Geometry check sheet. Reference: the model listing, model coordinates, mm. Coordinates: 2 decimals unless noted, no trailing zeros. Write each loop counter-clockwise with the first axis right and the second up, starting at its lowest first coordinate (ties: lowest second). Pieces come first, ordered by that corner, then holes. Notation, with made-up numbers: (-18.75, 76) -> (9.25, 76) arc R23 cw to (9.25, 102) -> close; hole circle Ø8 at (23.25, 11). An arc over 180 degrees is marked (long way). Put each result on its own line as item: value. Start each with the question number.
from build123d import *

# Parameters (mm, degrees)
F0_W        = 152.4
F0_H        = 101.6
F0_R        = 25.4
F1_DEPTH    = 76.2
F2_R        = 5.08
F3_R        = 5.08
F4_T1_DEPTH = 83.82
F4_S5_W     = 5.08
F4_S5_H     = 5.08
F4_T6_DEPTH = 5.08


# Not quite as in the source:
# - a fillet or chamfer that OpenCascade refuses, or shapes differently, is made with other operations: its cross-section is extruded or revolved along the edge and cut away or added


with BuildPart() as f1:
    # F0 (on Top) → F1 (new body)
    with BuildSketch(Plane.XY):
        Rectangle(F0_W, F0_H)
        Circle(F0_R, mode=Mode.SUBTRACT)
    extrude(amount=F1_DEPTH)

    # F2
    f2_edges = [f1.edges().sort_by_distance(p)[0] for p in [
        (-76.2, 0, 76.2),
    ]]
    fillet(f2_edges, radius=F2_R)

    # F3
    f3_edges = [f1.edges().sort_by_distance(p)[0] for p in [
        (2.54, 50.8, 76.2),
        (76.2, 0, 76.2),
        (2.54, -50.8, 76.2),
    ]]
    fillet(f3_edges, radius=F3_R)

    # F4: fillet of radius 5.08 on 1 edges, made by hand

    # F4_s2 → F4_t1 (cut)
    with BuildSketch(Plane.XY.offset(-12.7)):
        with BuildLine():
            ThreePointArc((76.2, -45.72), (74.7121024484, -49.3121024484), (71.12, -50.8))
            Line((71.12, -50.8), (76.2, -50.8))
            Line((76.2, -50.8), (76.2, -45.72))
        make_face()
    extrude(amount=F4_T1_DEPTH, mode=Mode.SUBTRACT)


with BuildPart() as f4_tool4:
    # F4_s5 → F4_t6 (new body)
    with BuildSketch(Plane.YZ.offset(71.12)):
        with Locations((-48.26, 73.66)):
            Rectangle(F4_S5_W, F4_S5_H)
    extrude(amount=F4_T6_DEPTH)

    # F4_s7 → F4_t8 (revolve, cut)
    with BuildSketch(Plane(origin=(71.12, -45.72, 71.12), x_dir=(0, 0.7071067812, -0.7071067812), z_dir=(0, -0.7071067812, -0.7071067812))):
        with BuildLine():
            ThreePointArc((0, -5.08), (5.08, 0), (0, 5.08))
            Line((0, 5.08), (0, -5.08))
        make_face()
    revolve(axis=Axis((71.12, -45.72, 71.12), (1, 0, 0)), mode=Mode.SUBTRACT)


with BuildPart() as f1_1:
    add(f1.part)

    # F4_t3: cut F4_tool4
    add(f4_tool4.part, mode=Mode.SUBTRACT)


solid = f1_1.part
Item 1: Section check A-A, the plane z = 37. Enter the section's corners in (x, y).
Item 2: Scan lines: line 1 along Y through (x, z) = (0, 47.5); line 2 along Y through (x, z) = (-13, 50); line 3 along X through (y, z) = (11.5, 53). Record each from-to range of solid material in increasing order. Write a range as [from, to].
Item 3: Section check C-C, the plane x = 0. Enter the section's corners in (y, z).
Item 4: Mould release check, pull along X, two halves, no side actions. Record for faces 1 (the flat face through (-76.2, -1, 35)), 2 (the flat face through (76.2, 2, 35)), 3 (the flat face through (-1, -50.8, 35)), 4 (the cylindrical face through (-5.506, -24.796, 37.567)): released by +X, released by -X, zero draft, split by the parting line, or undercut.
Item 5: Section check B-B, the plane y = 0. Enter the section's corners in (x, z), and give its area (3 significant figures).
From the geometry:
1. outline: (-76.2, -45.72) arc R5.08 ccw to (-71.12, -50.8) -> (71.12, -50.8) arc R5.08 ccw to (76.2, -45.72) -> (76.2, 50.8) -> (-71.12, 50.8) arc R5.08 ccw to (-76.2, 45.72) -> close; hole circle Ø50.8 at (0, 0)
2. line 1: [-50.8, -25.4], [25.4, 50.8]
2. line 2: [-50.8, -21.82], [21.82, 50.8]
2. line 3: [-76.2, -22.65], [22.65, 76.2]
3. outline: (-50.8, 0) -> (-25.4, 0) -> (-25.4, 76.2) -> (-45.72, 76.2) arc R5.08 ccw to (-50.8, 71.12) -> close; (25.4, 0) -> (50.8, 0) -> (50.8, 71.12) arc R5.08 ccw to (45.72, 76.2) -> (25.4, 76.2) -> close
4. face 1: released by -X
4. face 2: released by +X
4. face 3: zero draft
4. face 4: undercut
5. outline: (-76.2, 0) -> (-25.4, 0) -> (-25.4, 76.2) -> (-71.12, 76.2) arc R5.08 ccw to (-76.2, 71.12) -> close; (25.4, 0) -> (76.2, 0) -> (76.2, 71.12) arc R5.08 ccw to (71.12, 76.2) -> (25.4, 76.2) -> close
5. area: 7,730 mm²
